Autodesk Inventor part; units mm, degrees
ref_plane "YZ Plane" through (0, 0, 0) normal (1, 0, 0) x (0, 1, 0)
ref_plane "XZ Plane" through (0, 0, 0) normal (0, 1, 0) x (-1, 0, 0)
ref_plane "XY Plane" through (0, 0, 0) normal (0, 0, 1) x (1, 0, 0)
sketch "Sketch1" plane through (0, 0, 0) normal (1, 0, 0) x (0, 1, 0)
  line L0 (0, -6.7778) -> (70, -6.7778)
  line L1 (70, -6.7778) -> (70, -64.7778)
  line L2 (0, -64.7778) -> (0, -6.7778)
  line L3 (77, -64.7778) -> (77, 0.2222)
  line L4 (77, 0.2222) -> (-7, 0.2222)
  line L5 (-7, 0.2222) -> (-7, -64.7778)
  line L6 (-7, -64.7778) -> (77, -64.7778)
  point P0 (0, 0)
  dimension "d2" = 7
  dimension "d3" = 65
  dimension "d5" = 58
  dimension "d6" = 84
revolve "Revolution1" add sketch "Sketch1" angle 180 about axis through (0, -7, -64.7778) along (0, 1, 0) contours L2 L6 L5 L4 L3 L1 L0
sketch "Sketch2" plane through (0, -7, 0.2222) normal (-1, 0, 0) x (0, 0, 1)
  line L0 (0, 0) -> (-130, 0)
  line L1 (0, 0) -> (-130, 0)
  line L2 (0, 84) -> (0, 0)
  line L3 (0, 84) -> (-130, 84)
  line L4 (-130, 84) -> (-130, 0)
  line L5 (-7, 7) -> (-123, 7)
  line L6 (-123, 7) -> (-123, 77)
  line L7 (-7, 77) -> (-123, 77)
  line L8 (-7, 7) -> (-7, 77)
  line L9 (0, 0) -> (-42, 0)
  line L10 (-42, 0) -> (-42, 7)
  line L11 (-42, 7) -> (0, 7)
  line L12 (0, 7) -> (0, 0)
  line L13 (0, 0) -> (0, 42)
  line L14 (0, 77) -> (0, 84)
  point P0 (-0.2222, 7)
  point P1 (-130, 84)
  dimension "d7" = 42
extrude "Extrusion1" add sketch "Sketch2" along normal blind 110 contours L0 L10 L5 L11 L2
sketch "Sketch3" plane through (-110, -7, 0.2222) normal (0, -1, 0) x (1, 0, 0)
  line L0 (110, -42) -> (110, -130)
  arc A0 (110, -130) -> (110, 0) centre (110, -65) ccw
  line L1 (110, 0) -> (0, 0)
  line L2 (0, -42) -> (0, 0)
  line L3 (110, -42) -> (0, -42)
  line L4 (110, 0) -> (0, 0)
  line L5 (110, 0) -> (0, 0)
  line L6 (110, -42) -> (80, -42)
  line L7 (110, -42) -> (0, -42)
  line L8 (0, -42) -> (0, 0)
  line L9 (80, -42) -> (0, -22.0538)
  point P0 (110, -0.2222)
  dimension "d11" = 30
  dimension "d13" = 14
extrude "Extrusion2" cut sketch "Sketch3" against normal through all contours L3 L2 L9
ref_plane "Work Plane1" through (-110, 35, 0.2222) normal (0, -1, 0) x (1, 0, 0)
mirror "Mirror1" about plane through (-110, 35, 0.2222) normal (0, -1, 0) of "Extrusion1", "Extrusion2"
sketch "Sketch4" plane through (-110, -7, 0.2222) normal (0, -1, 0) x (1, 0, 0)
  line L0 (0, -22.0538) -> (80, -42)
  line L1 (110, -42) -> (80, -42)
  line L2 (110, -42) -> (110, -130)
  arc A0 (110, -130) -> (110, 0) centre (110, -65) ccw
  line L3 (110, 0) -> (0, 0)
  line L4 (0, -22.0538) -> (0, 0)
  line L5 (110, -84) -> (110, -42)
  line L6 (113, -65) -> (113, -44)
  line L7 (113, -44) -> (110, -44)
  line L8 (110, -44) -> (110, -65)
  line L9 (110, -86) -> (110, -42)
  line L10 (113, -65) -> (113, -86)
  line L11 (113, -86) -> (110, -86)
  line L12 (110, -44) -> (110, -86)
  line L13 (110, -42) -> (110, -123)
  point P0 (110, -0.2222)
  point P1 (110, -88)
  dimension "d17" = 21
  dimension "d18" = 3
extrude "Extrusion3" cut sketch "Sketch4" against normal through all contours L7 L6 L10 L11 L2
sketch "Sketch5" plane through (-110, -7, 0.2222) normal (0, -1, 0) x (1, 0, 0)
  line L0 (113, -86) -> (110, -86)
  line L1 (110, -86) -> (110, -130)
  arc A0 (110, -130) -> (110, 0) centre (110, -65) ccw
  line L2 (110, 0) -> (0, 0)
  line L3 (0, -22.0538) -> (0, 0)
  line L4 (0, -22.0538) -> (80, -42)
  line L5 (110, -42) -> (80, -42)
  line L6 (110, -42) -> (110, -44)
  line L7 (110, -44) -> (113, -44)
  line L8 (113, -44) -> (113, -86)
  line L9 (110, -130) -> (55.2127, -188.2954)
  arc A1 (110, -123) -> (110, -7) centre (110, -65) ccw
  line L10 (110, -123) -> (51.7311, -185)
  line L11 (51.7311, -185) -> (55.2244, -188.283)
  point P0 (110, -0.2222)
  dimension "d21" = 80
extrude "Extrusion4" add sketch "Sketch5" against normal blind 84 contours L1 L9 L11 L10
sketch "Sketch6" plane through (-110, -7, 0.2222) normal (0, -1, 0) x (1, 0, 0)
  line L0 (113, -86) -> (110, -86)
  line L1 (110, -86) -> (110, -123)
  line L2 (110, -123) -> (51.7311, -185)
  line L3 (51.7311, -185) -> (55.2244, -188.283)
  line L4 (55.2244, -188.283) -> (110, -130)
  arc A0 (110, -130) -> (110, 0) centre (110, -65) ccw
  line L5 (110, 0) -> (0, 0)
  line L6 (0, -22.0538) -> (0, 0)
  line L7 (0, -22.0538) -> (80, -42)
  line L8 (110, -42) -> (80, -42)
  line L9 (110, -42) -> (110, -44)
  line L10 (110, -44) -> (113, -44)
  line L11 (113, -44) -> (113, -86)
  line L12 (110, -65) -> (80, -65)
  line L13 (0, -107.9462) -> (80, -88)
  line L14 (110, -88) -> (80, -88)
  line L15 (0, -107.9462) -> (0, -185)
  line L16 (0, -185) -> (51.7311, -185)
  line L17 (110, -88) -> (110, -123)
  line L18 (110, -123) -> (51.7311, -185)
  point P0 (110, -0.2222)
extrude "Extrusion5" add sketch "Sketch6" against normal blind 7 contours L1 L2 L16 L15 L13 L14
mirror "Mirror2" about plane through (-110, 35, 0.2222) normal (0, -1, 0) of "Extrusion5"
sketch "Sketch7" plane through (-110, 77, 0.2222) normal (0, 1, 0) x (1, 0, 0)
  line L0 (0, 0) -> (68, 0)
  line L1 (110, 0) -> (0, 0)
  line L2 (68, 0) -> (68, 9)
  line L3 (68, 9) -> (0, 9)
  line L4 (0, 9) -> (0, 0)
  point P0 (110, 0.2222)
  dimension "d26" = 68
  dimension "d27" = 9
extrude "Extrusion6" cut sketch "Sketch7" against normal blind 84
properties part number "casco-salida-0,1"
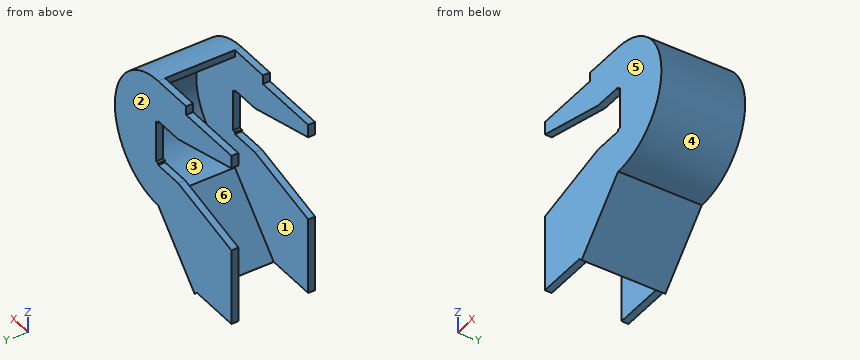
Here's how the part is built. I have some questions about the finished solid (model axes, mm). Face numbers are marked on the shaded views. A direction names the side the tool comes from. Give positions to 0.01 mm unless a question says otherwise; leave off trailing zeros. Order: outer loops, then holes, each group sorted by start corner. A loop starts at its lowest first (then second) coordinate and runs counter-clockwise, first axis right, second up. Notation, with made-up numbers: (57, 83.5) - (61, 83.5) arc R26 ccw to (61, 110.5) - close; hole circle Ø11 at (-36, -15.75). An arc over 180 degrees is marked (long way). Answer as a JSON object with one key per item and string values. Group by question number.
Item 1: For P1, Ø0.6, axis at y = -3, z = -87, coming from the -X side; P2, Ø7.5, axis at x = -16, y = 74.5, coming from the -Z side; P3, Ø10, axis at y = 55.5, z = -90, coming from the -X side, each with a flat end and sliding along its axis, tell me the tip position at first contact or that it passes through.
Item 2: If we section it at A-A on x = 53: Please give me the cut outline in (y, z), and give its area (3 significant figures).
Item 3: If we section it at C-C on z = -94.5: Please give me the cut outline in (x, y).
Item 4: Please list where these lines run through material, in increasing order: probe 1 along Y at (x, z) = (-40, -140.5); probe 2 along Z at (x, y) = (20.5, 66); probe 3 along Z at (x, y) = (3, 50).
Item 5: If we section it at D-D on x = -79: Please give me the cut outline in (y, z), and give its area (3 significant figures).
Item 6: Which directions (+Z, -Z, +X, -X, +Y, -Y) give clear straight access to the entire face, cutting with the end or side of a thin tool? Please do the marked faces 1 and 2.
Item 7: If we section it at B-B on y = 32.5: Please give me the cut outline in (x, z), and give its area (3 significant figures).
Item 8: If we mould it in two halves opening along Z, with no side actions, what happens to the marked faces 3, 4, 5 and 6? For each: pulls with the +Z half, pulls with the -Z half, needs draft (parallel to the pull), parting line crosses it, or undercut.
Result set:
{
 "1": {"P1": "x = 0", "P2": "z = -150.79", "P3": "x = 49.5"},
 "2": {"outline": "(-7, -102.41) - (77, -102.41) - (77, -27.15) - (-7, -27.15) - close; hole (0, -88.34) - (70, -88.34) - (70, -41.22) - (0, -41.22) - close", "area": "3,020 mm²"},
 "3": {"outline": "(-56.96, -7) - (57.81, -7) - (57.81, 77) - (-56.96, 77) - (-56.96, 70) - (49.81, 70) - (49.81, 0) - (-56.96, 0) - close"},
 "4": {"probe 1": "-7 to 0, 70 to 77", "probe 2": "-126.46 to -119.03, -10.52 to -3.1", "probe 3": "-129.71 to -122.7, -6.86 to 0.15"},
 "5": {"outline": "(-7, -184.78) - (0, -184.78) - (0, -99.99) - (-7, -99.99) - close; (-7, -29.56) - (0, -29.56) - (0, -8.78) - (-7, -8.78) - close; (70, -184.78) - (77, -184.78) - (77, -99.99) - (70, -99.99) - close; (70, -29.56) - (77, -29.56) - (77, -8.78) - (70, -8.78) - close", "area": "1,480 mm²"},
 "6": {"face 1": "-X", "face 2": "+Z, -Z, +X, -X, +Y"},
 "7": {"outline": "(-58.27, -184.78) - (-54.78, -188.06) - (0, -129.78) arc R65 ccw to (0, 0.22) - (0, -6.78) arc R58 cw to (0, -122.78) - close", "area": "1,750 mm²"},
 "8": {"face 3": "undercut", "face 4": "parting line crosses it", "face 5": "needs draft", "face 6": "pulls with the +Z half"}
}
